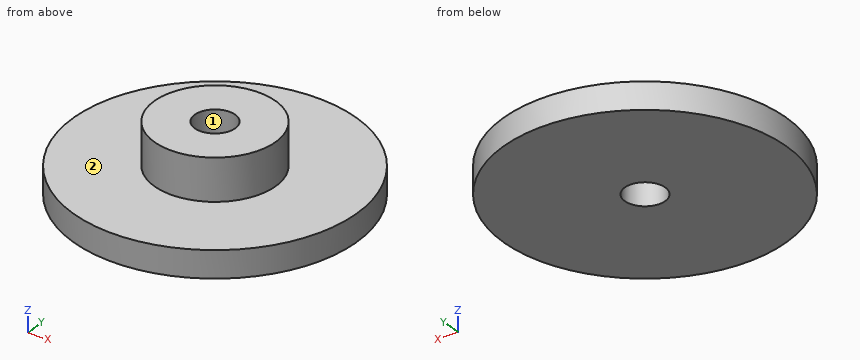
from build123d import *

# Parameters (mm, degrees)
CROQUIS1_R              = 10.5
SALIENTE_EXTRUIR1_DEPTH = 2
CROQUIS2_R              = 4.5
SALIENTE_EXTRUIR2_DEPTH = 3.1
CORTAR_EXTRUIR1_REACH   = 17.701
CROQUIS3_R              = 1.5


with BuildPart() as part:
    # Croquis1 → Saliente-Extruir1 (new body)
    with BuildSketch(Plane.XY):
        Circle(CROQUIS1_R)
    extrude(amount=SALIENTE_EXTRUIR1_DEPTH)

    # Croquis2 → Saliente-Extruir2 (add)
    with BuildSketch(Plane.XY.offset(2)):
        with Locations(Location((0, 0, 0), (0, 0, 180))):
            Circle(CROQUIS2_R)
    extrude(amount=SALIENTE_EXTRUIR2_DEPTH)

    # Croquis3 → Cortar-Extruir1 (cut, up to next)
    with BuildSketch(Plane.XY.offset(5.1), mode=Mode.PRIVATE) as cortar_extruir1_sk1:
        Circle(CROQUIS3_R)
    cortar_extruir1_tool1 = extrude(cortar_extruir1_sk1.sketch, amount=-CORTAR_EXTRUIR1_REACH, mode=Mode.PRIVATE) & part.part
    add(cortar_extruir1_tool1.solids().sort_by_distance((0, 0, 5.1))[0], mode=Mode.SUBTRACT)


solid = part.part
Could you check a few things on this model? Use its own coordinates, in mm. Face numbers are marked on the shaded views. A direction names the side the tool comes from. Give positions to 0.01 mm unless a question says otherwise; leave off trailing zeros. Loops run counter-clockwise (first coordinate to the right, second up) from the corner with the lowest first, then second, coordinate; pieces in that order, holes last. Notation, with made-up numbers: (-13, -36.5) -> (15, -36.5) arc R29 cw to (15, -8.5) -> close; hole circle Ø9 at (-39, 76). An arc over 180 degrees is marked (long way). Return JSON: item names as keys, results as strings.
Item 1: I need wall thicknesses on L1, parallel to Y at x = 0, z = 1.15; L2, parallel to Y at x = 0, z = 2.1; L3, parallel to Z at x = 3.5, y = 9.25. Which ranges of each line are inside material? Lowest first, please. Write a range as from..to.
Geometry results:
{"L1": "y = -10.5..-1.5, 1.5..10.5", "L2": "y = -4.5..-1.5, 1.5..4.5", "L3": "z = 0..2"}
Item 2: If we section it at D-D on y = 2.25: List the corners of the cut face in (x, z) for me.
Geometry results:
{"outline": "(-10.26, 0) -> (10.26, 0) -> (10.26, 2) -> (3.9, 2) -> (3.9, 5.1) -> (-3.9, 5.1) -> (-3.9, 2) -> (-10.26, 2) -> close"}
Item 3: I'm going to push flat-ended pins straight in: pin 1 (1 mm diameter, centred on y = 4.5, z = 4.5, fed in from +X); pin 2 (2 mm diameter, centred on x = -5, y = 5.5, fed in from +Z); pin 3 (1 mm diameter, centred on y = 4, z = 3, fed in from +X). Where does each tip first touch, or does it pass through?
Geometry results:
{"pin 1": "stops at x = 2.06", "pin 2": "stops at z = 2", "pin 3": "stops at x = 2.83"}
Item 4: Which directions (+Z, -Z, +X, -X, +Y, -Y) give clear straight access to the entire face, cutting with the end or side of a thin tool? Please do the marked faces 1 and 2.
Geometry results:
{"face 1": "+Z, -Z", "face 2": "+Z"}
Item 5: If we section it at A-A on y = 0: List the corners of the cut face in (x, z) for me.
Geometry results:
{"outline": "(-10.5, 0) -> (-1.5, 0) -> (-1.5, 5.1) -> (-4.5, 5.1) -> (-4.5, 2) -> (-10.5, 2) -> close; (1.5, 0) -> (10.5, 0) -> (10.5, 2) -> (4.5, 2) -> (4.5, 5.1) -> (1.5, 5.1) -> close"}
Item 6: If we section it at C-C on z = 0.8: List the corners of the cut face in (x, y) for me.
Geometry results:
{"outline": "circle Ø21 at (0, 0); hole circle Ø3 at (0, 0)"}
